Drawing for the job (mm, zero at the part's lowest x, y, z). Coordinates: 2 decimals unless noted, no trailing zeros. Loops run counter-clockwise (first coordinate to the right, second up) from the corner with the lowest first, then second, coordinate; pieces in that order, holes last. Notation, with made-up numbers: (-21.5, 42) -> (31.5, 42) arc R11 ccw to (31.5, 63) -> close; hole circle Ø8 at (-37.5, -2.75). An arc over 180 degrees is marked (long way). Write item = value, one per line. Start each with the question number.
(1) Band-saw the part on C-C (z = 162). Write the cut outline in (x, y).
(2) Flat gauge pins, fed straight in: P1, Ø1.9, axis at x = 38.5, z = 38.5, coming from the +Y side; P2, Ø1, axis at x = 6, y = 8, coming from the +Z side; P3, Ø1.5, axis at y = 1.5, z = 195, coming from the -X side; P4, Ø1.5, axis at y = 4.5, z = 42.5, coming from the +X side. Where does each tip first touch, or does it go through?
(3) Band-saw the part on B-B (y = 8.5). Count the separate pieces of the cut face and the enclosed holes in it, and give its area (3 significant figures).
(4) Drill centre lines: line 1 (X direction, y = 2.25, z = 23); line 2 (X direction, y = 4, z = 38.5); line 3 (Z direction, x = 22.5, y = 7). Where is each one in solid material? Low to high. Write a range as from..to.
(5) Band-saw the part on A-A (x = 27.5). Write the cut outline in (y, z), and give its area (3 significant figures).
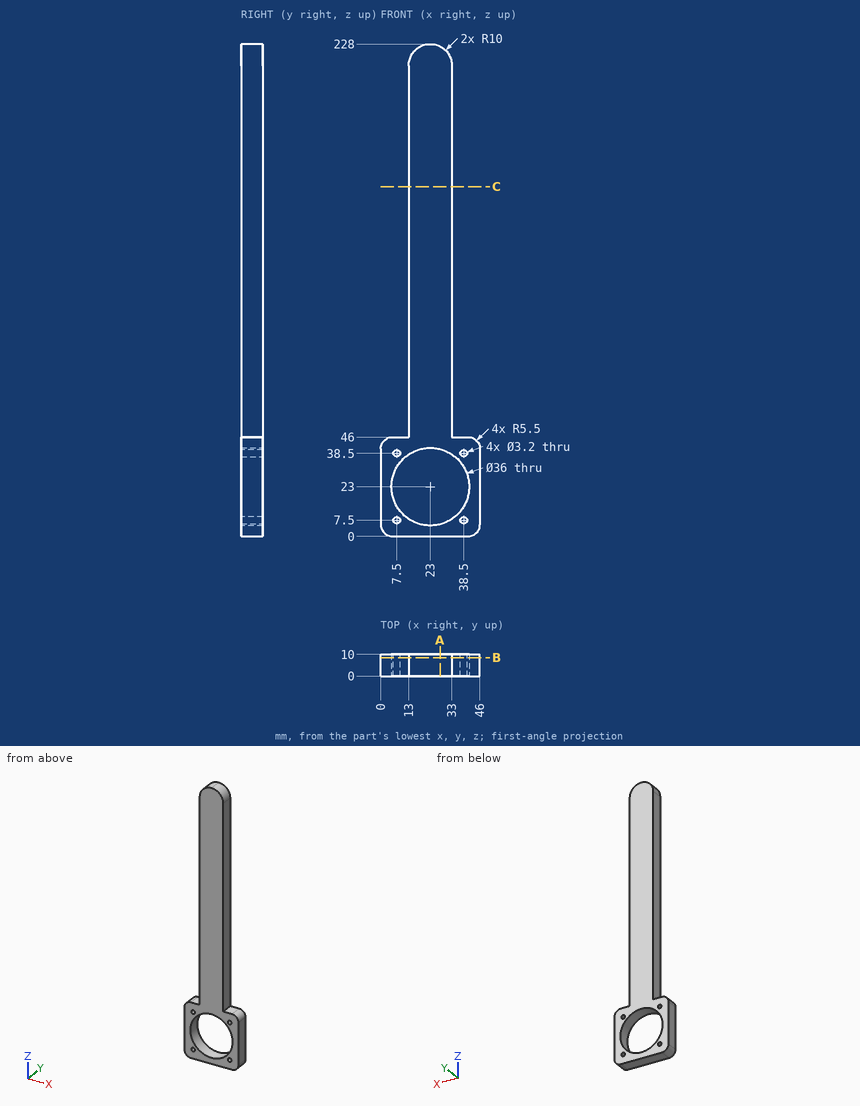
Findings below:
q1.outline = (13, 0) -> (33, 0) -> (33, 10) -> (13, 10) -> close
q2.P1 = through
q2.P2 = 46
q2.P3 = 13
q2.P4 = 45.86
q3.separate_pieces = 1
q3.enclosed_holes = 5
q3.area = 4,640 mm²
q4.line_1 = 0..5, 41..46
q4.line_2 = 0..5.9, 9.1..13.85, 32.15..36.9, 40.1..46
q4.line_3 = 0..5.01, 40.99..227.99
q5.outline = (0, 0) -> (10, 0) -> (10, 5.57) -> (0, 5.57) -> close; (0, 40.43) -> (10, 40.43) -> (10, 226.93) -> (0, 226.93) -> close
q5.area = 1,920 mm²
